The listing builds one solid part. Answer for the finished solid, in the listing's coordinates (mm). A direction names the side the tool comes from. Coordinates: 2 decimals unless noted, no trailing zeros. Loops run counter-clockwise (first coordinate to the right, second up) from the corner with the lowest first, then second, coordinate; pieces in that order, holes last. Notation, with made-up numbers: (-32, 48.25) - (-7, 48.25) arc R30 cw to (-7, 84.25) - close; hole circle Ø6 at (11.5, 67.25). An arc over 180 degrees is marked (long way). Put each result on its own line as item: value.
```python
from build123d import *

# Parameters (mm, degrees)
ESQUISSE1_W                  = 55
ESQUISSE1_H                  = 42.3
BOSS_EXTRU_1_DEPTH           = 25.5
ESQUISSE4_R                  = 18.1
ENL_V_MAT_EXTRU_3_DEPTH      = 22.5
ENL_V_MAT_EXTRU_4_DEPTH      = 62.713369702
ENL_V_MAT_EXTRU_4_DEPTH_BACK = 62.713369702
ESQUISSE5_R                  = 11
ESQUISSE6_R                  = 1.625
ENL_V_MAT_EXTRU_5_DEPTH      = 10
BOSS_EXTRU_2_DEPTH           = 40
ESQUISSE16_W                 = 5.5
ESQUISSE16_H                 = 10.832527472
BOSS_EXTRU_4_DEPTH           = 14.5


with BuildPart() as part:
    # Esquisse1 → Boss.-Extru.1 (new body)
    with BuildSketch(Plane.XY):
        with Locations((27.5, 21.15)):
            Rectangle(ESQUISSE1_W, ESQUISSE1_H)
    extrude(amount=BOSS_EXTRU_1_DEPTH)

    # Esquisse4 → Enlèv. mat.-Extru.3 (cut)
    with BuildSketch(Plane.XY):
        with Locations(Location((27.5, 21.15, 0), (0, 0, 180))):
            Circle(ESQUISSE4_R)
    extrude(amount=ENL_V_MAT_EXTRU_3_DEPTH, mode=Mode.SUBTRACT)

    # Esquisse5 → Enlèv. mat.-Extru.4 (cut, two sides: drawn at the far end of the back side and taken through both)
    with BuildSketch(Plane(origin=(37, 0, 25.5), x_dir=(-1, 0, 0), z_dir=(0, 0, -1)).offset(-ENL_V_MAT_EXTRU_4_DEPTH_BACK)):
        with Locations((9.5, 21.15)):
            Circle(ESQUISSE5_R)
    extrude(amount=ENL_V_MAT_EXTRU_4_DEPTH + ENL_V_MAT_EXTRU_4_DEPTH_BACK, mode=Mode.SUBTRACT)

    # Esquisse6 → Enlèv. mat.-Extru.5 (cut)
    with BuildSketch(Plane(origin=(0, 0, 25.5), x_dir=(-1, 0, 0), z_dir=(0, 0, -1))):
        with Locations((-37.399494937, 31.049494937)):
            Circle(ESQUISSE6_R)
        with Locations((-17.600505063, 31.049494937)):
            Circle(ESQUISSE6_R)
        with Locations((-17.600505063, 11.250505063)):
            Circle(ESQUISSE6_R)
        with Locations((-37.399494937, 11.250505063)):
            Circle(ESQUISSE6_R)
    extrude(amount=ENL_V_MAT_EXTRU_5_DEPTH, mode=Mode.SUBTRACT)

    # Esquisse7 → Boss.-Extru.2 (add)
    with BuildSketch(Plane.XY.offset(25.5)):
        Polygon((55, 0), (73, 0), (73, 5), (58.367411306, 5), (55, 10.832527472), align=None)
        Polygon((-18, 0), (-18, 5), (-3.367411306, 5), (0, 10.832527472), (0, 0), align=None)
    extrude(amount=-BOSS_EXTRU_2_DEPTH)

    # Esquisse16 → Boss.-Extru.4 (add)
    with BuildSketch(Plane(origin=(0, 0, 0), x_dir=(-1, 0, 0), z_dir=(0, 0, -1))):
        with Locations((-2.75, 5.416263736)):
            Rectangle(ESQUISSE16_W, ESQUISSE16_H)
        with Locations((-52.25, 5.416263736)):
            Rectangle(ESQUISSE16_W, ESQUISSE16_H)
    extrude(amount=BOSS_EXTRU_4_DEPTH)


solid = part.part
```
1) The part is cut by section C-C (z = 21.5). Give the vertices of the cut face in (x, y).
Found:
outline: (-18, 0) - (73, 0) - (73, 5) - (58.37, 5) - (55, 10.83) - (55, 42.3) - (0, 42.3) - (0, 10.83) - (-3.37, 5) - (-18, 5) - close; hole circle Ø36.2 at (27.5, 21.15)
2) For a pull along Y with two mould halves and no side action, classify faces 1 (the face through (5.5, 5, -7)), 2 (the face through (16.85, 9.81, 24.02)), 3 (the face through (-1.707, 7.875, 5.78)), 4 (the face through (28, 0, 10)) as pulls with the +Y half, pulls with the -Y half, needs draft (parallel to the pull), parting line crosses it, or undercut.
Found:
face 1: needs draft
face 2: undercut
face 3: pulls with the +Y half
face 4: pulls with the -Y half
3) The part is cut by section A-A (y = 21.15). Give the vertices of the cut face in (x, z).
Found:
outline: (0, 0) - (9.4, 0) - (9.4, 22.5) - (16.5, 22.5) - (16.5, 25.5) - (0, 25.5) - close; (38.5, 22.5) - (45.6, 22.5) - (45.6, 0) - (55, 0) - (55, 25.5) - (38.5, 25.5) - close
4) Straight lines are drawn through the part: L1, parallel to Z at x = 48, y = 3; L2, parallel to X at y = 21, z = 24; L3, parallel to Y at x = 40.5, z = 18. For each, find the intervals that lie inside material, in ascending order. Write a range as [from, to].
Found:
L1: z = [0, 25.5]
L2: x = [0, 16.5], [38.5, 55]
L3: y = [0, 8.56], [33.74, 42.3]
5) Each of these flat-tipped pins is pushed along its axis until it touches: pin 1 (2.5 mm diameter, centred on x = 17.6, y = 11.25, fed in from -Z); pin 2 (21 mm diameter, centred on x = 28, y = 25, fed in from -Z); pin 3 (4 mm diameter, centred on y = 7.5, z = 21, fed in from +X); pin 4 (6 mm diameter, centred on x = 3, z = -6, fed in from +Y). Where does it stop, or does it pass through?
Found:
pin 1: passes through
pin 2: stops at z = 22.5
pin 3: stops at x = 58.08
pin 4: stops at y = 10.83
6) The part is cut by section B-B (x = 27.5). Give the vertices of the cut face in (y, z), and give its area (3 significant figures).
Found:
outline: (0, 0) - (3.05, 0) - (3.05, 22.5) - (10.15, 22.5) - (10.15, 25.5) - (0, 25.5) - close; (32.15, 22.5) - (39.25, 22.5) - (39.25, 0) - (42.3, 0) - (42.3, 25.5) - (32.15, 25.5) - close
area: 198 mm^2
7) The part is cut by section D-D (x = 51). Give the vertices of the cut face in (y, z).
Found:
outline: (0, -14.5) - (10.83, -14.5) - (10.83, 0) - (42.3, 0) - (42.3, 25.5) - (0, 25.5) - close
8) For faces 5 (the face through (0, 26, 13)), 6 (the face through (55, 26, 13)), 7 (the face through (49.5, 5, -7)), 8 (the face through (52, 10.833, -7)), determine the directions among +Z, -Z, +X, -X, +Y, -Y from which every point of the face is accessible in a straight line to the end or side of a thin tool.
Found:
face 5: +Z, -Z, -X, +Y
face 6: +Z, -Z, +X, +Y
face 7: -Z, +Y, -Y
face 8: -Z, +X, -X, +Y
